from build123d import *

# Parameters (mm, degrees)
SKETCH1_R           = 2.25
SKETCH1_R_2         = 5
BOSS_EXTRUDE1_DEPTH = 4
FILLET1_R           = 15
SKETCH2_R           = 7.5
SKETCH2_R_2         = 2.25
BOSS_EXTRUDE2_DEPTH = 2


with BuildPart() as part:
    # Sketch1 → Boss-Extrude1 (new body)
    with BuildSketch(Plane(origin=(0, 0, 0), x_dir=(1, 0, 0), z_dir=(0, 1, 0))):
        with BuildLine():
            ThreePointArc((-5, -69.409830056), (0, -82.5), (5, -69.409830056))
            Line((5, -69.409830056), (5, 69.409830056))
            ThreePointArc((5, 69.409830056), (0, 82.5), (-5, 69.409830056))
            Line((-5, 69.409830056), (-5, -69.409830056))
        make_face()
        with Locations(Location((0, -75, 0), (0, 0, 270))):
            Circle(SKETCH1_R, mode=Mode.SUBTRACT)
        with Locations(Location((0, 75, 0), (0, 0, 270))):
            Circle(SKETCH1_R_2, mode=Mode.SUBTRACT)
    extrude(amount=BOSS_EXTRUDE1_DEPTH)

    # Fillet1
    fillet1_edges = [part.edges().sort_by_distance(p)[0] for p in [
        (-5, 2, 69.409830056),
        (-5, 2, -69.409830056),
        (5, 2, -69.409830056),
        (5, 2, 69.409830056),
    ]]
    fillet(fillet1_edges, radius=FILLET1_R)

    # Sketch2 → Boss-Extrude2 (add)
    with BuildSketch(Plane(origin=(0, 4, 0), x_dir=(1, 0, 0), z_dir=(0, 1, 0))):
        with Locations(Location((0, -75, 0), (0, 0, 27.266044451))):
            Circle(SKETCH2_R)
        with Locations(Location((0, -75, 0), (0, 0, 270))):
            Circle(SKETCH2_R_2, mode=Mode.SUBTRACT)
    extrude(amount=BOSS_EXTRUDE2_DEPTH)


solid = part.part
Build history of the part. All positions in model axes, mm. A direction names the side the tool comes from. Coordinates: 2 decimals unless noted, no trailing zeros. Write each loop counter-clockwise with the first axis right and the second up, starting at its lowest first coordinate (ties: lowest second). Pieces come first, ordered by that corner, then holes.
(1) Cut at C-C on z = 75. List the corners of the cut face in (x, y), and give its area (3 significant figures).
(2) Pin check, flat tips, straight feed: pin 1 Ø2 at (y, z) = (4.5, 25.5) entering from -X; pin 2 Ø3 at (x, y) = (-6, 1) entering from +Z; pin 3 Ø2 at (x, y) = (1.5, 2) entering from +Z. Stop position of each tip, or through.
(3) Drill centre lines: line 1 (Z direction, x = 1.75, y = 2.65); line 2 (Z direction, x = 1, y = 2); line 3 (Y direction, x = -1.5, z = 0.5). Where is each one in solid material? Low to high.
(4) Cut at A-A on x = 0. List the corners of the cut face in (y, z), and give its area (3 significant figures).
(5) Cut at D-D on z = -75. List the corners of the cut face in (x, y).
(6) Mould opens along X. For faces 1 (the cylindrical face through (0.215, 1.972, -82.497)), 2 (the flat face through (-2.4, 6, 74.2)), 3 (the cylindrical face through (-1.915, 1.972, -70.381)), 4 (the flat face through (5, 2, 1)) say: pulls with the +X half, pulls with the -X half, needs draft (parallel to the pull), parting line crosses it, or undercut.
(7) Cut at B-B on y = 1.45. List the corners of the cut face in (x, z), and give its area (3 significant figures).
(8) 3-axis set-ups, long thin cutter, end or side, ignore diameter. For faces 5 (the cylindrical face through (5.41, 2.03, -68.18)), 6 (the flat face through (-5, 2, -1)), 7 (the flat face through (0, 0, -1)): which of +Z, -Z, +X, -X, +Y, -Y reach the whole face in a straight line?
Working result:
1. outline: (-7.5, 0) - (-2.25, 0) - (-2.25, 6) - (-7.5, 6) - close; (2.25, 0) - (7.5, 0) - (7.5, 6) - (2.25, 6) - close
1. area: 63.0 mm2
2. pin 1: stops at x = -5
2. pin 2: stops at z = 81
2. pin 3: stops at z = 82.48
3. line 1: z = -82.29 to -79.68, -70.32 to 73.59, 76.41 to 82.29
3. line 2: z = -82.43 to -79.9, -70.1 to 72.98, 77.02 to 82.43
3. line 3: y = 0 to 4
4. outline: (0, -82.5) - (4, -82.5) - (4, -80) - (0, -80) - close; (0, -70) - (4, -70) - (4, 67.5) - (6, 67.5) - (6, 72.75) - (0, 72.75) - close; (0, 77.25) - (6, 77.25) - (6, 82.5) - (0, 82.5) - close
4. area: 623 mm2
5. outline: (-7.5, 0) - (-5, 0) - (-5, 4) - (-7.5, 4) - close; (5, 0) - (7.5, 0) - (7.5, 4) - (5, 4) - close
6. face 1: parting line crosses it
6. face 2: needs draft
6. face 3: undercut
6. face 4: pulls with the +X half
7. outline: (-6.67, -71.56) arc R7.5 ccw (long way) to (6.67, -71.56) arc R15 cw to (5, -64.69) - (5, 64.69) arc R15 cw to (6.67, 71.56) arc R7.5 ccw (long way) to (-6.67, 71.56) arc R15 cw to (-5, 64.69) - (-5, -64.69) arc R15 cw to start; hole circle Ø10 at (0, -75); hole circle Ø4.5 at (0, 75)
7. area: 1,630 mm2
8. face 5: +X, +Y, -Y
8. face 6: -X, +Y, -Y
8. face 7: +Z, -Z, +X, -X, -Y
